CAD build for the part. Positions are in the model's coordinates, mm. Round coordinates to 2 decimals unless told otherwise and drop trailing zeros. Order: outer loops, then holes, each group sorted by start corner. A loop starts at its lowest first (then second) coordinate and runs counter-clockwise, first axis right, second up. Notation, with made-up numbers: (25.25, 22.5) -> (29.25, 22.5) arc R19 cw to (29.25, 57.5) -> close; hole circle Ø5 at (-23.75, 48.5). An arc over 180 degrees is marked (long way). Return JSON: item names as keys, results as strings. Group by question number.
Q1. Probe line 1 along X through (y, z) = (-0.3, 0); line 2 along Z through (x, y) = (0.25, -0.5) (3 decimals); line 3 along Z through (x, y) = (1, -0.65). List the from-to ranges inside material, lowest first.
Q2. Cut at A-A (z = 0). Write the cut outline in (x, y).
Q3. Cut at C-C (y = -0.2). Write the cut outline in (x, z), then the cut area to 3 significant figures.
Q4. Cut at D-D (z = -4.5). Write the cut outline in (x, y).
Q5. Cut at B-B (x = 0). Write the cut outline in (y, z), then the cut area to 4 significant figures.
from build123d import *

# Parameters (mm, degrees)
SKETCH1_R          = 6.25
BASE_FLANGE1_DEPTH = 0.7
SKETCH4_W          = 1
SKETCH4_H          = 3.25
CUT_EXTRUDE1_DEPTH = 0.7
SKETCH5_R          = 1.7
CUT_EXTRUDE2_DEPTH = 0.7


# Sheet-metal steps are written as plain solids
with BuildPart() as part:
    # Sketch1 → Base-Flange1 (new body)
    with BuildSketch(Plane(origin=(0, 0, 0), x_dir=(1, 0, 0), z_dir=(0, 1, 0))):
        with Locations(Location((0, 0, 0), (0, 0, 270))):
            Circle(SKETCH1_R)
    extrude(amount=-BASE_FLANGE1_DEPTH)

    # Sketch4 → Cut-Extrude1 (cut)
    with BuildSketch(Plane(origin=(0, 0, 0), x_dir=(1, 0, 0), z_dir=(0, 1, 0))):
        with Locations((0, -4.625)):
            Rectangle(SKETCH4_W, SKETCH4_H)
    extrude(amount=-CUT_EXTRUDE1_DEPTH, mode=Mode.SUBTRACT)

    # Sketch5 → Cut-Extrude2 (cut)
    with BuildSketch(Plane(origin=(0, 0, 0), x_dir=(1, 0, 0), z_dir=(0, 1, 0))):
        with Locations(Location((0, 0, 0), (0, 0, 270))):
            Circle(SKETCH5_R)
    extrude(amount=-CUT_EXTRUDE2_DEPTH, mode=Mode.SUBTRACT)


solid = part.part
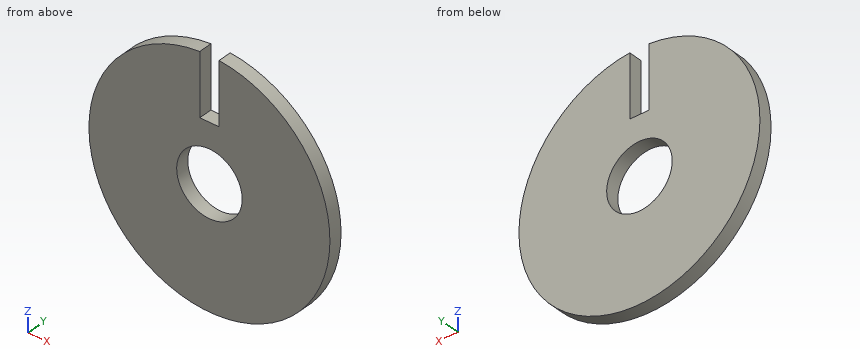
Solution:
{
 "1": {"line 1": "x = -6.25 to -1.7, 1.7 to 6.25", "line 2": "z = -6.245 to -1.682, 1.682 to 3", "line 3": "z = -6.17 to -1.37, 1.37 to 6.17"},
 "2": {"outline": "(-6.25, -0.7) -> (-1.7, -0.7) -> (-1.7, 0) -> (-6.25, 0) -> close; (1.7, -0.7) -> (6.25, -0.7) -> (6.25, 0) -> (1.7, 0) -> close"},
 "3": {"outline": "(-0.5, 3) -> (-0.5, 6.23) arc R6.25 ccw (long way) to (0.5, 6.23) -> (0.5, 3) -> close; hole circle Ø3.4 at (0, 0)", "area": "110 mm²"},
 "4": {"outline": "(-4.34, -0.7) -> (4.34, -0.7) -> (4.34, 0) -> (-4.34, 0) -> close"},
 "5": {"outline": "(-0.7, -6.25) -> (0, -6.25) -> (0, -1.7) -> (-0.7, -1.7) -> close; (-0.7, 1.7) -> (0, 1.7) -> (0, 3) -> (-0.7, 3) -> close", "area": "4.095 mm²"}
}
